The model under review builds one solid part; all positions refer to its coordinate system, in mm. Give positions to 0.01 mm unless a question says otherwise; leave off trailing zeros. Loops run counter-clockwise (first coordinate to the right, second up) from the corner with the lowest first, then second, coordinate; pieces in that order, holes last. Notation, with made-up numbers: M -12.75,25.5 L 42.25,25.5 A13 cw 42.25,47.5 Z; hole C -16.5,64 d6. An arc over 180 degrees is marked long. Write item = value, one per line. Start each with the question number.
1. For pin 1 (4 mm diameter, centred on x = -88.5, z = -97.5, fed in from +Y); pin 2 (4 mm diameter, centred on x = -51.5, z = -63.5, fed in from -Y); pin 3 (8 mm diameter, centred on x = -23.5, z = -45, fed in from +Y); pin 4 (3 mm diameter, centred on x = -67.5, z = -108, fed in from +Y), all flat-tipped, find the tip position at first contact; note any pin that passes through.
2. Wall thickness on line 1 along X through (y, z) = (270, -34.5); line 2 along X through (y, z) = (320.5, -21.5); line 3 along Y through (x, z) = (-86, -17): over which ranges is each line inside the solid? List them lowest first. Write a range as from..to.
3. We need section A-A on z = -89.5. Give the boundary of the cut face in (x, y).
4. We need section B-B on x = -46. Give the boundary of the cut face in (y, z).
Autodesk Inventor part; units mm, degrees
ref_plane "Work Plane1" through (0, 381, 0) normal (-0.766, -0.6428, 0) x (0, 0, -1)
ref_plane "YZ Plane" through (0, 0, 0) normal (1, 0, 0) x (0, 1, 0)
ref_plane "XZ Plane" through (0, 0, 0) normal (0, 1, 0) x (-1, 0, 0)
sketch "Sketch1" plane through (0, 0, 0) normal (0, 1, 0) x (-1, 0, 0)
  line L0 (0, 0) -> (127, 0)
  line L1 (127, 0) -> (127, -127)
  line L2 (127, -127) -> (0, -127)
  line L3 (0, -127) -> (0, 0)
  dimension "d0" = 127
  dimension "d1" = 127
extrude "Extrusion1" add sketch "Sketch1" along normal blind 254
sketch "Sketch2" plane through (0, 254, 0) normal (0, 1, 0) x (1, 0, 0)
  line L0 (-127, 0) -> (0, 0)
  line L1 (-127, 127) -> (-127, 0)
  line L2 (0, 0) -> (-127, 0)
  line L3 (-127, 0) -> (-127, 127)
  line L4 (-127, 127) -> (0, 127)
  line L5 (0, 127) -> (0, 0)
extrude "Extrusion2" add sketch "Sketch2" along normal blind 127
ref_plane "Work Plane1" through (0, 381, 0) normal (-0.766, -0.6428, 0) x (0, 0, -1)
sketch "Sketch4" plane through (0, 381, 0) normal (-0.766, -0.6428, 0) x (0, 0, -1)
  line L0 (-9.5876, -147.9681) -> (139.0202, -147.9681)
  line L1 (139.0202, -147.9681) -> (139.0202, 162.4304)
  line L2 (139.0202, 162.4304) -> (-9.5876, 162.4304)
  line L3 (-9.5876, 162.4304) -> (-9.5876, -147.9681)
  point P0 (0, 291.8629)
extrude "Extrusion3" cut sketch "Sketch4" along normal blind 127
sketch "Sketch6" plane through (-97.2876, 299.366, 0) normal (0.766, 0.6428, 0) x (0, 0, -1)
  line L0 (127, -151.3527) -> (0, -151.3527)
  line L1 (0, 46.2242) -> (127, 46.2242)
  line L2 (0, -151.3527) -> (127, -151.3527)
  line L3 (127, -151.3527) -> (127, 46.2242)
  line L4 (127, 46.2242) -> (0, 46.2242)
  line L5 (0, 46.2242) -> (0, -151.3527)
  point P0 (0, -291.8629)
properties part number "NestArmP2-ver1-1111-2021"
Final values:
q1.pin_1 = 291.27
q1.pin_2 = 0
q1.pin_3 = 216.19
q1.pin_4 = 265.65
q2.line_1 = -127..-72.65
q2.line_2 = -127..-115.02
q2.line_3 = 0..285.91
q3.outline = M -127,0 L 0,0 L 0,183.42 L -127,334.77 Z
q4.outline = M 0,-127 L 238.24,-127 L 238.24,0 L 0,0 Z
